Autodesk Inventor part; units mm, degrees
ref_plane "YZ Plane" through (0, 0, 0) normal (1, 0, 0) x (0, 1, 0)
ref_plane "XZ Plane" through (0, 0, 0) normal (0, 1, 0) x (-1, 0, 0)
ref_plane "XY Plane" through (0, 0, 0) normal (0, 0, 1) x (1, 0, 0)
sketch "Эскиз1" plane through (0, 0, 0) normal (0, 0, 1) x (1, 0, 0)
  circle A0 centre (0, 0) radius 75
  circle A1 centre (0, 0) radius 34
  dimension "d0" = 150
  dimension "d1" = 68
extrude "Выдавливание1" add sketch "Эскиз1" along normal blind 10
sketch "Эскиз2" plane through (0, 0, 10) normal (0, 0, 1) x (1, 0, 0)
  circle A0 centre (-64, 0) radius 4
  point P0 (0, 0)
  dimension "d4" = 8
  dimension "d5" = 64
extrude "Выдавливание2" cut sketch "Эскиз2" against normal blind 12
pattern_circular "Круговой массив1" count 2 over 360 about axis through (0, 0, 0) along (0, 0, 1) of "Выдавливание2"
sketch "Эскиз3" plane through (0, 0, 0) normal (0, 1, 0) x (-1, 0, 0)
  line L0 (0, 0) -> (0, 5)
  dimension "d32" = 5
hole "Отверстие1" at (0, 0, 5) direction (0, 1, 0) diameter 4.9 end through all counterbore diameter 5 counterbore depth 75.455
sketch "Эскиз4" plane through (0, 0, 0) normal (0, 0, -1) x (-1, 0, 0)
  circle A0 centre (0, 0) radius 34
  line L0 (0, -34) -> (0, -67)
  circle A1 centre (0, -67) radius 2
  dimension "d18" = 33
  dimension "d33" = 4
extrude "Выдавливание3" cut sketch "Эскиз4" against normal blind 12 contours A1
sketch "Эскиз6" plane through (0, 0, 0) normal (0, 0, -1) x (-1, 0, 0)
  line L0 (0, 0) -> (0, 67)
  circle A0 centre (0, 67) radius 2
  dimension "d34" = 67
  dimension "d35" = 4
extrude "Выдавливание5" cut sketch "Эскиз6" against normal blind 5
sketch "Эскиз7" plane through (0, 0, 0) normal (0, 0, -1) x (-1, 0, 0)
  circle A0 centre (64, 0) radius 4
  circle A1 centre (-64, 0) radius 4
  circle A2 centre (64, 0) radius 5
  circle A3 centre (-64, 0) radius 5
  point P0 (0, 0)
  dimension "d38" = 10
  dimension "d39" = 10
extrude "Выдавливание6" cut sketch "Эскиз7" against normal blind 1
sketch "Эскиз8" plane through (0, 0, 0) normal (0, 0, -1) x (-1, 0, 0)
  circle A0 centre (32.5, 56.2917) radius 1.5
  circle A1 centre (11.2871, -64.0125) radius 1.5
  circle A2 centre (-41.7812, 49.7929) radius 1.5
  point P0 (0, 0)
extrude "Выдавливание7" cut sketch "Эскиз8" against normal through all
sketch "Эскиз9" plane through (0, 0, 0) normal (0, 0, -1) x (-1, 0, 0)
  circle A0 centre (0, 0) radius 53
  circle A1 centre (0, 0) radius 55
  dimension "d44" = 106
  dimension "d45" = 110
extrude "Выдавливание8" cut sketch "Эскиз9" against normal blind 1.5
properties part number "В сальник" material "Чугун, серый"
Model file for the job. Use its own axes, mm. A direction names the side the tool comes from. Give positions to 0.01 mm unless a question says otherwise; leave off trailing zeros. Write each loop counter-clockwise with the first axis right and the second up, starting at its lowest first coordinate (ties: lowest second). Pieces come first, ordered by that corner, then holes. Notation, with made-up numbers: (61, -24.75) - (76, -24.75) arc R17 ccw to (76, -8.75) - close; hole circle Ø9 at (61.25, 87.25). An arc over 180 degrees is marked (long way). Answer as CSV lines item,"result".
1. Two-plate mould, pull along X, no slides. Class faces 1 (the face through (68.995, 0.22, 0.493)), 2 (the face through (-9.764, -74.362, 4.93)), 3 (the face through (35, 1, 0)): +X half, -X half, draft (parallel to the pull), parting line (faces both ways), or undercut.
Responses:
face 1,"undercut"
face 2,"parting line"
face 3,"draft"
2. Band-saw the part on B-B (y = -2). Count the separate pieces of the cut face and the enclosed holes in it, and give its area (3 significant figures).
Responses:
separate pieces,"4"
enclosed holes,"0"
area,"672 mm2"
3. Band-saw the part on C-C (x = -64). Write the cut outline in (y, z).
Responses:
outline,"(-39.1, 0) - (-5, 0) - (-5, 1) - (-4, 1) - (-4, 10) - (-39.1, 10) - close; (4, 1) - (5, 1) - (5, 0) - (39.1, 0) - (39.1, 10) - (4, 10) - close"
4. Band-saw the part on A-A (x = 0). Write the cut outline in (y, z).
Responses:
outline,"(-75, 0) - (-69, 0) - (-69, 10) - (-75, 10) - close; (-65, 0) - (-55, 0) - (-55, 1.5) - (-53, 1.5) - (-53, 0) - (-34, 0) - (-34, 10) - (-65, 10) - close; (34, 0) - (53, 0) - (53, 1.5) - (55, 1.5) - (55, 0) - (65, 0) - (65, 2.5) - (34, 2.5) - close; (34, 7.5) - (75, 7.5) - (75, 10) - (34, 10) - close; (69, 0) - (75, 0) - (75, 2.5) - (69, 2.5) - close"
5. Pin check, flat tips, straight feed: pin 1 (4 mm diameter, centred on x = -4, z = 5, fed in from +Y); pin 2 (3 mm diameter, centred on x = 6, z = 1, fed in from -Y); pin 3 (1.5 mm diameter, centred on y = -13.5, z = 7.5, fed in from +X). Stop position of each tip, or through.
Responses:
pin 1,"stops at y = 74.97"
pin 2,"stops at y = -74.86"
pin 3,"stops at x = 73.91"
6. Band-saw the part on D-D (y = -49.5). Write the cut outline in (x, z), and give its area (3 significant figures).
Responses:
outline,"(-56.34, 0) - (-23.97, 0) - (-23.97, 1.5) - (-18.94, 1.5) - (-18.94, 0) - (18.94, 0) - (18.94, 1.5) - (23.97, 1.5) - (23.97, 0) - (56.34, 0) - (56.34, 10) - (-56.34, 10) - close"
area,"1,110 mm2"
7. 3-axis set-ups, long thin cutter, end or side, ignore diameter. For faces 4 (the face through (0, -65, 5)), 5 (the face through (-1.908, 67.601, 1.337)), 6 (the face through (-0.1, 54.7, 7.5)): which of +Z, -Z, +X, -X, +Y, -Y reach the whole face in a straight line?
Responses:
face 4,"+Z, -Z"
face 5,"-Z"
face 6,"+Y"
8. Drill centre lines: L1, parallel to Y at x = 0, z = 0.9; L2, parallel to X at y = 30, z = 0.75; L3, parallel to Y at x = -24, z = 0.75. Where is each one in solid material? Low to high. Write a range as [from, to].
Responses:
L1,"y = [-75, -69], [-65, -55], [-53, -34], [34, 53], [55, 65], [69, 75]"
L2,"x = [-68.74, -46.1], [-43.69, -16], [16, 43.69], [46.1, 68.74]"
L3,"y = [-71.06, -49.49], [-47.25, -24.08], [24.08, 47.25], [49.49, 71.06]"
